Autodesk Inventor part; units mm, degrees
ref_plane "YZ Plane" through (0, 0, 0) normal (1, 0, 0) x (0, 1, 0)
ref_plane "XZ Plane" through (0, 0, 0) normal (0, 1, 0) x (-1, 0, 0)
ref_plane "XY Plane" through (0, 0, 0) normal (0, 0, 1) x (1, 0, 0)
sketch "Sketch1" plane through (0, 0, 0) normal (0, 0, 1) x (1, 0, 0)
  line L0 (-9, -13.5) -> (9, -13.5)
  line L1 (13.5, -9) -> (13.5, 9)
  line L2 (9, 13.5) -> (-9, 13.5)
  line L3 (-13.5, 9) -> (-13.5, -9)
  line L4 (-13.5, -13.5) -> (13.5, 13.5) construction
  line L5 (13.5, -13.5) -> (-13.5, 13.5) construction
  line L6 (-8, -8) -> (8, -8) construction
  line L7 (8, -8) -> (8, 8) construction
  line L8 (8, 8) -> (-8, 8) construction
  line L9 (-8, 8) -> (-8, -8) construction
  line L10 (-8, -8) -> (8, 8) construction
  line L11 (8, -8) -> (-8, 8) construction
  circle A0 centre (-8, 8) radius 1.5
  circle A1 centre (8, 8) radius 1.5
  circle A2 centre (-8, -8) radius 1.5
  circle A3 centre (8, -8) radius 1.5
  arc A4 (-9, 13.5) -> (-13.5, 9) centre (-9, 9) ccw
  arc A5 (-13.5, -9) -> (-9, -13.5) centre (-9, -9) ccw
  arc A6 (9, -13.5) -> (13.5, -9) centre (9, -9) ccw
  arc A7 (13.5, 9) -> (9, 13.5) centre (9, 9) ccw
  circle A8 centre (0, 0) radius 4.925
  dimension "d0" = 27
  dimension "d1" = 27
  dimension "d2" = 16
  dimension "d3" = 16
  dimension "d4" = 3
  dimension "d5" = 3
  dimension "d6" = 3
  dimension "d7" = 3
  dimension "d8" = 4.5
  dimension "d9" = 9.85
extrude "Extrusion1" add sketch "Sketch1" along normal blind 3.7
properties part number "Tope_rodamiento" material "PMMA Plastic"
Verification items for the finished model (mm, model axes). Round coordinates to 2 decimals unless told otherwise and drop trailing zeros. Write each loop counter-clockwise with the first axis right and the second up, starting at its lowest first coordinate (ties: lowest second). Pieces come first, ordered by that corner, then holes.
(1) Material ranges on line 1 (Y direction, x = -8, z = 1.15); line 2 (X direction, y = 0.25, z = 2.2); line 3 (Y direction, x = 0, z = 1.45) (3 decimals), recorded low to high.
Returned:
line 1: y = -13.5 to -9.5, -6.5 to 6.5, 9.5 to 13.5
line 2: x = -13.5 to -4.92, 4.92 to 13.5
line 3: y = -13.5 to -4.925, 4.925 to 13.5
(2) Section check C-C (z = 0.85). Enter the section's corners in (x, y) (3 decimals).
Returned:
outline: (-13.5, -9) arc R4.5 ccw to (-9, -13.5) - (9, -13.5) arc R4.5 ccw to (13.5, -9) - (13.5, 9) arc R4.5 ccw to (9, 13.5) - (-9, 13.5) arc R4.5 ccw to (-13.5, 9) - close; hole circle Ø3 at (-8, -8); hole circle Ø3 at (-8, 8); hole circle Ø9.85 at (0, 0); hole circle Ø3 at (8, -8); hole circle Ø3 at (8, 8)
(3) Depth check by flat-ended pin: pin 1 Ø1 at (y, z) = (10, 3) entering from +X; pin 2 Ø2.5 at (x, y) = (8, 8) entering from -Z. Enter the tip coordinate at first touch or a pass-through.
Returned:
pin 1: stops at x = 13.47
pin 2: passes through
(4) Section check D-D (x = 8). Enter the section's corners in (y, z), plus the area to 3 significant figures.
Returned:
outline: (-13.5, 0) - (-9.5, 0) - (-9.5, 3.7) - (-13.5, 3.7) - close; (-6.5, 0) - (6.5, 0) - (6.5, 3.7) - (-6.5, 3.7) - close; (9.5, 0) - (13.5, 0) - (13.5, 3.7) - (9.5, 3.7) - close
area: 77.7 mm2
(5) Section check A-A (y = 0). Enter the section's corners in (x, z) (3 decimals).
Returned:
outline: (-13.5, 0) - (-4.925, 0) - (-4.925, 3.7) - (-13.5, 3.7) - close; (4.925, 0) - (13.5, 0) - (13.5, 3.7) - (4.925, 3.7) - close
